Verification items for the finished model (mm, model axes). Face numbers are marked on the shaded views. A direction names the side the tool comes from. Round coordinates to 2 decimals unless told otherwise and drop trailing zeros. Loops run counter-clockwise (first coordinate to the right, second up) from the corner with the lowest first, then second, coordinate; pieces in that order, holes last. Notation, with made-up numbers: (7, 70) -> (62, 70) arc R21 ccw to (62, 77) -> close; hole circle Ø4 at (-27, -36). An arc over 180 degrees is marked (long way). Use CSV: the item, a comma, the result in double quotes. Start each with the question number.
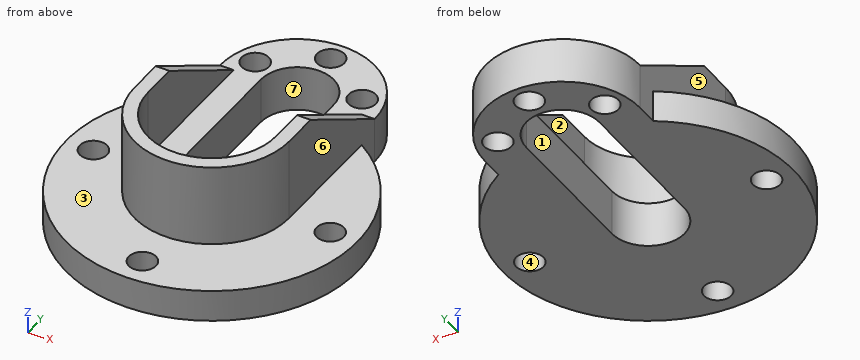
```python
from build123d import *

# Parameters (mm, degrees)
SKETCH1_R           = 4.7625
BOSS_EXTRUDE1_DEPTH = 11.1125
SKETCH1_3_R         = 4.7625
BOSS_EXTRUDE2_DEPTH = 15.875
BOSS_EXTRUDE3_DEPTH = 39.6875
CUT_EXTRUDE1_DEPTH  = 78.7875


with BuildPart() as part:
    # Sketch1 → Boss-Extrude1 (new body)
    with BuildSketch(Plane.XY):
        with BuildLine():
            Line((26.9875, 43.038527435), (26.9875, 0))
            ThreePointArc((26.9875, 0), (0, -26.9875), (-26.9875, 0))
            Line((-26.9875, 0), (-26.9875, 43.038527435))
            ThreePointArc((-26.9875, 43.038527435), (0, -50.8), (26.9875, 43.038527435))
        make_face()
        with Locations((0, -41.275)):
            Circle(SKETCH1_R, mode=Mode.SUBTRACT)
        with Locations((-41.275, 0)):
            Circle(SKETCH1_R, mode=Mode.SUBTRACT)
        with Locations((41.275, 0)):
            Circle(SKETCH1_R, mode=Mode.SUBTRACT)
        with BuildLine():
            ThreePointArc((-22.225, 0), (0, -22.225), (22.225, 0))
            Line((22.225, 0), (22.225, 50.8))
            Line((22.225, 50.8), (26.9875, 50.8))
            Line((26.9875, 50.8), (26.9875, 0))
            ThreePointArc((26.9875, 0), (0, -26.9875), (-26.9875, 0))
            Line((-26.9875, 0), (-26.9875, 50.8))
            Line((-26.9875, 50.8), (-22.225, 50.8))
            Line((-22.225, 50.8), (-22.225, 0))
        make_face()
        with BuildLine():
            Line((-22.225, 0), (-22.225, 50.8))
            Line((-22.225, 50.8), (-26.9875, 50.8))
            ThreePointArc((-26.9875, 50.8), (0, 77.7875), (26.9875, 50.8))
            Line((26.9875, 50.8), (22.225, 50.8))
            Line((22.225, 50.8), (22.225, 0))
            ThreePointArc((22.225, 0), (0, -22.225), (-22.225, 0))
        make_face()
        with Locations((-18.647025444, 57.586962219)):
            Circle(SKETCH1_R, mode=Mode.SUBTRACT)
        with Locations((0, 70.64375)):
            Circle(SKETCH1_R, mode=Mode.SUBTRACT)
        with Locations((18.647025444, 57.586962219)):
            Circle(SKETCH1_R, mode=Mode.SUBTRACT)
        with BuildLine():
            ThreePointArc((-12.7, 0), (0, -12.7), (12.7, 0))
            Line((12.7, 0), (12.7, 50.8))
            ThreePointArc((12.7, 50.8), (0, 63.5), (-12.7, 50.8))
            Line((-12.7, 50.8), (-12.7, 0))
        make_face(mode=Mode.SUBTRACT)
    extrude(amount=BOSS_EXTRUDE1_DEPTH)

    # Sketch1_3 → Boss-Extrude2 (add)
    with BuildSketch(Plane.XY):
        with BuildLine():
            ThreePointArc((-22.225, 0), (0, -22.225), (22.225, 0))
            Line((22.225, 0), (22.225, 50.8))
            Line((22.225, 50.8), (26.9875, 50.8))
            Line((26.9875, 50.8), (26.9875, 0))
            ThreePointArc((26.9875, 0), (0, -26.9875), (-26.9875, 0))
            Line((-26.9875, 0), (-26.9875, 50.8))
            Line((-26.9875, 50.8), (-22.225, 50.8))
            Line((-22.225, 50.8), (-22.225, 0))
        make_face()
        with BuildLine():
            Line((-22.225, 0), (-22.225, 50.8))
            Line((-22.225, 50.8), (-26.9875, 50.8))
            ThreePointArc((-26.9875, 50.8), (0, 77.7875), (26.9875, 50.8))
            Line((26.9875, 50.8), (22.225, 50.8))
            Line((22.225, 50.8), (22.225, 0))
            ThreePointArc((22.225, 0), (0, -22.225), (-22.225, 0))
        make_face()
        with Locations((-18.647025444, 57.586962219)):
            Circle(SKETCH1_3_R, mode=Mode.SUBTRACT)
        with Locations((0, 70.64375)):
            Circle(SKETCH1_3_R, mode=Mode.SUBTRACT)
        with Locations((18.647025444, 57.586962219)):
            Circle(SKETCH1_3_R, mode=Mode.SUBTRACT)
        with BuildLine():
            ThreePointArc((-12.7, 0), (0, -12.7), (12.7, 0))
            Line((12.7, 0), (12.7, 50.8))
            ThreePointArc((12.7, 50.8), (0, 63.5), (-12.7, 50.8))
            Line((-12.7, 50.8), (-12.7, 0))
        make_face(mode=Mode.SUBTRACT)
    extrude(amount=BOSS_EXTRUDE2_DEPTH)

    # Sketch1_4 → Boss-Extrude3 (add)
    with BuildSketch(Plane.XY):
        with BuildLine():
            ThreePointArc((-22.225, 0), (0, -22.225), (22.225, 0))
            Line((22.225, 0), (22.225, 50.8))
            Line((22.225, 50.8), (26.9875, 50.8))
            Line((26.9875, 50.8), (26.9875, 0))
            ThreePointArc((26.9875, 0), (0, -26.9875), (-26.9875, 0))
            Line((-26.9875, 0), (-26.9875, 50.8))
            Line((-26.9875, 50.8), (-22.225, 50.8))
            Line((-22.225, 50.8), (-22.225, 0))
        make_face()
    extrude(amount=BOSS_EXTRUDE3_DEPTH)

    # Sketch2 → Cut-Extrude1 (cut, through all)
    with BuildSketch(Plane(origin=(26.9875, 0, 0), x_dir=(0, 0, -1), z_dir=(1, 0, 0))):
        Polygon((-15.875, 50.8), (-39.6875, 12.7), (-39.6875, 50.8), align=None)
    extrude(amount=-CUT_EXTRUDE1_DEPTH, mode=Mode.SUBTRACT)


solid = part.part
```
Q1. Thickness scan on L1, parallel to X at y = 28.5, z = 17 (1 decimal); L2, parallel to X at y = 14, z = 15.5; L3, parallel to Z at x = -30.5, y = -33.5. Record the ranges inside material, lowest first. Write a range as from..to.
Q2. Release check for a two-part mould opening along X. For the marked faces 4, 5, 6 and 7 record: +X half, -X half, draft (parallel to the pull), parting line (faces both ways), or undercut.
Q3. Cross-section at A-A (x = 0). Record the boundary of the cut face in (y, z) (1 decimal), and give its area (3 significant figures).
Q4. Depth check by flat-ended pin: pin 1 Ø8 at (y, z) = (36, 4.5) entering from +X; pin 2 Ø10 at (y, z) = (45.5, 8) entering from -X; pin 3 Ø10 at (x, y) = (-3.5, 47) entering from -Z; pin 4 Ø2 at (y, z) = (-17.5, 6.5) entering from -X. Enter the tip coordinate at first touch or a pass-through.
Q5. Cross-section at C-C (x = -19.5). Record the boundary of the cut face in (y, z) (1 decimal), and give its area (3 significant figures).
Q6. Cross-section at B-B (y = 7.5). Record the boundary of the cut face in (x, z) (1 decimal).
Q7. Tool access check on the marked faces 1, 2 and 3. Record the directions out of +Z, -Z, +X, -X, +Y, -Y that give a thin tool (end or side, any length) a straight path to the whole face; none if there is none.
Answer list:
1,L1,"x = -27..-22.2, 22.2..27"
1,L2,"x = -26.99..-12.7, 12.7..26.99"
1,L3,"z = 0..11.11"
2,face 4,"undercut"
2,face 5,"-X half"
2,face 6,"+X half"
2,face 7,"undercut"
3,outline,"(-50.8, 0) -> (-46, 0) -> (-46, 11.1) -> (-50.8, 11.1) -> close; (-36.5, 0) -> (-12.7, 0) -> (-12.7, 15.9) -> (-22.2, 15.9) -> (-22.2, 39.7) -> (-27, 39.7) -> (-27, 11.1) -> (-36.5, 11.1) -> close; (63.5, 0) -> (65.9, 0) -> (65.9, 15.9) -> (63.5, 15.9) -> close; (75.4, 0) -> (77.8, 0) -> (77.8, 15.9) -> (75.4, 15.9) -> close"
3,area,"575 mm2"
4,pin 1,"stops at x = 39.45"
4,pin 2,"stops at x = -30.67"
4,pin 3,"passes through"
4,pin 4,"stops at x = -48.05"
5,outline,"(-46.9, 0) -> (52.9, 0) -> (52.9, 15.9) -> (-10.7, 15.9) -> (-10.7, 39.7) -> (-18.7, 39.7) -> (-18.7, 11.1) -> (-46.9, 11.1) -> close; (62.3, 0) -> (69.5, 0) -> (69.5, 15.9) -> (62.3, 15.9) -> close"
5,area,"1,750 mm2"
6,outline,"(-50.2, 0) -> (-12.7, 0) -> (-12.7, 15.9) -> (-22.2, 15.9) -> (-22.2, 39.7) -> (-27, 39.7) -> (-27, 11.1) -> (-50.2, 11.1) -> close; (12.7, 0) -> (50.2, 0) -> (50.2, 11.1) -> (27, 11.1) -> (27, 39.7) -> (22.2, 39.7) -> (22.2, 15.9) -> (12.7, 15.9) -> close"
7,face 1,"+Z, -Z"
7,face 2,"+Z, +Y"
7,face 3,"+Z, -Y"
